The listing builds one solid part. Answer for the finished solid, in the listing's coordinates (mm). A direction names the side the tool comes from. Round coordinates to 2 decimals unless told otherwise and drop trailing zeros. Write each loop counter-clockwise with the first axis right and the second up, starting at its lowest first coordinate (ties: lowest second). Pieces come first, ordered by that corner, then holes. Notation, with made-up numbers: (-24.75, 34.25) - (-10.75, 34.25) arc R17 ccw to (-10.75, 38.25) - close; hole circle Ø8 at (29.25, -26.75). An arc over 180 degrees is marked (long way). Use a Markdown table: item, result. Add a question column.
1) Find the intervals of material crossed by probe 1 along X at (y, z) = (1.3, 0); probe 2 along Z at (x, y) = (8, 0.7); probe 3 along X at (y, z) = (1, -2), in increasing order. Write a range as from..to.
2) Each of these flat-tipped pins is pushed along its axis until it touches: P1, Ø4, axis at x = 11.5, z = -0.5, coming from the -Y side; P2, Ø3, axis at x = 8.58, z = 0, coming from the -Y side; P3, Ø0.9, axis at x = 11.5, z = 3, coming from the -Y side; P4, Ø1.5, axis at y = 1.5, z = -2.5, coming from the +X side. Where does it stop, or does it pass through?
3) A tool of negligible diameter and unlimited length cuts with its end or side. For faces 1 (the flat face through (7, 3.2, -2)), 2 (the flat face through (5, 1, 6.7)), 3 (the cylindrical face through (9.872, 1.014, 2.024)), 4 (the flat face through (1, 0, -2)), 5 (the flat face through (15.282, 1, -6)), from which of +Z, -Z, +X, -X, +Y, -Y can it reach the whole face along a straight path? Write none if from no direction.
4) Determine the mould class of faces 6 (the flat face through (15.982, 2, -7)), 7 (the flat face through (8, 1, -6.7)), 8 (the flat face through (8, 2, -7.9)) for opening direction X: +X half, -X half, draft (parallel to the pull), parting line (faces both ways), or undercut.
5) A cutting plane is placed at D-D (z = 0). Give the vertices of the cut face in (x, y), then the cut area to 3 significant figures.
6) A cutting plane is placed at B-B (x = 4.75). Give the vertices of the cut face in (y, z), then the cut area to 3 significant figures.
7) A cutting plane is placed at A-A (y = 1.6). Give the vertices of the cut face in (x, z).
8) A cutting plane is placed at C-C (z = -6.25). Give the vertices of the cut face in (x, y).
```python
from build123d import *

# Parameters (mm, degrees)
MAINBASESKETCH_W          = 15.8
MAINBASESKETCH_H          = 3.2
MAINBASEEXTRUDE_DEPTH     = 7.9
MAINBASESHELL_T           = -1.2
UNDERSIDECIRCLEEXT_START  = -0.2
UNDERSIDECIRCLESKETCH_R   = 3.1
UNDERSIDECIRCLESKETCH_R_2 = 2.4
UNDERSIDECIRCLEEXT_DEPTH  = 2.2
ANGLEDCUT_DEPTH           = 19.555463972
CUT_EXTRUDE16_DEPTH       = 2.2


with BuildPart() as part:
    # MainBaseSketch → MainBaseExtrude (new, symmetric)
    with BuildSketch(Plane.XY):
        with Locations((8.581967213, 1.6)):
            Rectangle(MAINBASESKETCH_W, MAINBASESKETCH_H)
    extrude(amount=MAINBASEEXTRUDE_DEPTH, both=True)

    # MainBaseShell
    mainbaseshell_openings = [part.faces().sort_by_distance(p)[0] for p in [
        (8.581967213, 0, 0),
    ]]
    offset(amount=MAINBASESHELL_T, openings=mainbaseshell_openings, kind=Kind.INTERSECTION)

    # UnderSideCircleSketch → UnderSideCircleExt (add)
    with BuildSketch(Plane.XZ.offset(-2).offset(UNDERSIDECIRCLEEXT_START)):
        with Locations((8.581967213, 0)):
            Circle(UNDERSIDECIRCLESKETCH_R)
        with Locations((8.581967213, 0)):
            Circle(UNDERSIDECIRCLESKETCH_R_2, mode=Mode.SUBTRACT)
    extrude(amount=UNDERSIDECIRCLEEXT_DEPTH)

    # AngledCutSketch → AngledCut (cut, through all)
    with BuildSketch(Plane.XZ):
        Polygon((8.7465188, 7.575344166), (15.981967213, -6.7), (15.981967213, -7.9), (16.481967213, -7.9), (16.481967213, 7.9), (8.581967213, 7.9), align=None)
    extrude(amount=-ANGLEDCUT_DEPTH, mode=Mode.SUBTRACT)

    # AngledNotchSketch → Cut-Extrude16 (cut)
    with BuildSketch(Plane(origin=(0, 0, 0), x_dir=(-1, 0, 0), z_dir=(0, -1, 0))):
        with BuildLine():
            Line((-10.711153505, -3.699172992), (-11.897271127, -1.358994981))
            ThreePointArc((-11.897271127, -1.358994981), (-11.034832221, -2.39254887), (-10.711153505, -3.699172992))
        make_face()
    extrude(amount=-CUT_EXTRUDE16_DEPTH, mode=Mode.SUBTRACT)


solid = part.part
```
Entries:
| question | item | result |
|---|---|---|
| 1 | probe 1 | x = 0.68..1.88, 5.48..6.18, 10.98..11.68 |
| 1 | probe 2 | z = -7.9..-6.7, -3.04..-2.33, 2.33..3.04, 6.7..7.9 |
| 1 | probe 3 | x = 0.68..1.88, 6.21..7.26, 9.91..10.95 |
| 2 | P1 | stops at y = 0 |
| 2 | P2 | stops at y = 2 |
| 2 | P3 | stops at y = 2.2 |
| 2 | P4 | stops at x = 14.14 |
| 3 | face 1 | +Z, -Z, +X, -X, +Y |
| 3 | face 2 | +X, -Y |
| 3 | face 3 | -Y |
| 3 | face 4 | +Z, -Z, +X, -X, -Y |
| 3 | face 5 | +Z, -Y |
| 4 | face 6 | +X half |
| 4 | face 7 | undercut |
| 4 | face 8 | draft |
| 5 | outline | (0.68, 0) - (1.88, 0) - (1.88, 2) - (5.48, 2) - (5.48, 0) - (6.18, 0) - (6.18, 2) - (10.98, 2) - (10.98, 0) - (11.68, 0) - (11.68, 2) - (12.59, 2) - (12.59, 3.2) - (0.68, 3.2) - close |
| 5 | area | 19.5 mm² |
| 6 | outline | (0, -7.9) - (3.2, -7.9) - (3.2, 7.9) - (0, 7.9) - (0, 6.7) - (2, 6.7) - (2, -6.7) - (0, -6.7) - close |
| 6 | area | 23.8 mm² |
| 7 | outline | (0.68, -7.9) - (15.98, -7.9) - (15.98, -6.7) - (15.28, -5.32) - (15.28, -6.7) - (1.88, -6.7) - (1.88, 6.7) - (9.19, 6.7) - (8.58, 7.9) - (0.68, 7.9) - close; circle Ø6.2 at (8.58, 0); hole circle Ø4.8 at (8.58, 0) |
| 8 | outline | (0.68, 0) - (1.88, 0) - (1.88, 2) - (15.28, 2) - (15.28, 0) - (15.75, 0) - (15.75, 3.2) - (0.68, 3.2) - close |
